The listing builds one solid part. Answer for the finished solid, in the listing's coordinates (mm). A direction names the side the tool comes from. Give positions to 0.01 mm unless a question says otherwise; leave off trailing zeros. Write each loop counter-clockwise with the first axis right and the second up, starting at its lowest first coordinate (ties: lowest second). Pieces come first, ordered by that corner, then holes. Notation, with made-up numbers: (33.25, 35.25) - (78.25, 35.25) arc R21 ccw to (78.25, 41.25) - close; hole circle Ø11 at (50, 20). An arc over 180 degrees is marked (long way). One line per question, with ' | ' between items. Start each with the question number.
1. The mould has two halves that part along X. Classify faces 1 (the face through (9.84, 20.28, -0.08)), 2 (the face through (3.175, 16, 0)), 3 (the face through (-6, 10.795, 0)): +X half, -X half, draft (parallel to the pull), parting line (faces both ways), or undercut.
2. A cutting plane is placed at B-B (y = 17.25). Determine the outline of the cut face in (x, z) (1 decimal), then the cut area to 3 significant figures.
3. For faces 4 (the face through (-2.09, 2.46, -3.83)), 5 (the face through (-15.24, 5, 5)), determine the directions among +Z, -Z, +X, -X, +Y, -Y from which every point of the face is accessible in a straight line to the end or side of a thin tool.
4. A cutting plane is placed at C-C (z = 0). Determine the outline of the cut face in (x, y) (1 decimal), then the cut area to 3 significant figures.
5. A cutting plane is placed at D-D (x = -11). Determine the outline of the cut face in (y, z) (1 decimal).
6. A cutting plane is placed at A-A (x = 11). Determine the outline of the cut face in (y, z).
7. Find the intervals of material crossed by L1, parallel to X at y = 15.75, z = -1.75 (3 decimals); L2, parallel to Y at x = -9.5, z = 0 (1 decimal); L3, parallel to Y at x = 9.5, z = 0.5, in increasing order. Write a range as from..to.
8. Given P1, Ø5.5, axis at x = -10, z = 2.5, coming from the +Y side (3 decimals); P2, Ø6, axis at y = 5, z = 0, coming from the -X side; P3, Ø1, axis at y = 16, z = -2, coming from the -X side (3 decimals), each flat-ended and moving along its own axis, determine where each tip first touches the part or whether it passes through.
```python
from build123d import *

# Parameters (mm, degrees)
SKETCH1_W           = 30.48
SKETCH1_H           = 10.795
BOSS_EXTRUDE1_DEPTH = 10.795
SKETCH2_R           = 4.826
CUT_EXTRUDE1_DEPTH  = 26.67
SKETCH3_W           = 12.065
SKETCH3_H           = 10.795
BOSS_EXTRUDE2_DEPTH = 10.795
SKETCH4_R           = 4.826
CUT_EXTRUDE2_DEPTH  = 25.4


with BuildPart() as part:
    # Sketch1 → Boss-Extrude1 (new body)
    with BuildSketch(Plane(origin=(0, 0, 0), x_dir=(1, 0, 0), z_dir=(0, 1, 0))):
        Rectangle(SKETCH1_W, SKETCH1_H)
    extrude(amount=BOSS_EXTRUDE1_DEPTH)

    # Sketch2 → Cut-Extrude1 (cut)
    with BuildSketch(Plane.ZY.offset(15.24)):
        with Locations((0, 5.3975)):
            Circle(SKETCH2_R)
    extrude(amount=-CUT_EXTRUDE1_DEPTH, mode=Mode.SUBTRACT)

    # Sketch3 → Boss-Extrude2 (add)
    with BuildSketch(Plane(origin=(0, 10.795, 0), x_dir=(1, 0, 0), z_dir=(0, 1, 0))):
        with Locations((9.2075, 0)):
            Rectangle(SKETCH3_W, SKETCH3_H)
    extrude(amount=BOSS_EXTRUDE2_DEPTH)

    # Sketch4 → Cut-Extrude2 (cut)
    with BuildSketch(Plane(origin=(0, 0, -5.3975), x_dir=(-1, 0, 0), z_dir=(0, 0, -1))):
        with Locations((-9.2075, 15.494)):
            Circle(SKETCH4_R)
    extrude(amount=-CUT_EXTRUDE2_DEPTH, mode=Mode.SUBTRACT)


solid = part.part
```
Determined:
1) face 1: undercut | face 2: -X half | face 3: draft
2) outline: (3.2, -5.4) - (4.7, -5.4) - (4.7, 5.4) - (3.2, 5.4) - close; (13.7, -5.4) - (15.2, -5.4) - (15.2, 5.4) - (13.7, 5.4) - close | area: 33.2 mm2
3) face 4: -X | face 5: +Z, -Z, -X, +Y, -Y
4) outline: (-15.2, 0) - (15.2, 0) - (15.2, 21.6) - (3.2, 21.6) - (3.2, 10.8) - (-15.2, 10.8) - (-15.2, 10.2) - (11.4, 10.2) - (11.4, 0.6) - (-15.2, 0.6) - close; hole circle Ø9.7 at (9.2, 15.5) | area: 129 mm2
5) outline: (0, -5.4) - (10.8, -5.4) - (10.8, 5.4) - (0, 5.4) - close; hole circle Ø9.7 at (5.4, 0)
6) outline: (0, -5.4) - (11.01, -5.4) - (11.01, 5.4) - (0, 5.4) - close; (19.97, -5.4) - (21.59, -5.4) - (21.59, 5.4) - (19.97, 5.4) - close; hole circle Ø9.65 at (5.4, 0)
7) L1: 3.175..4.388, 14.027..15.24 | L2: 0..0.6, 10.2..10.8 | L3: 0..0.6, 10.2..10.68, 20.31..21.59
8) P1: y = 10.795 | P2: x = 11.43 | P3: x = 3.175
